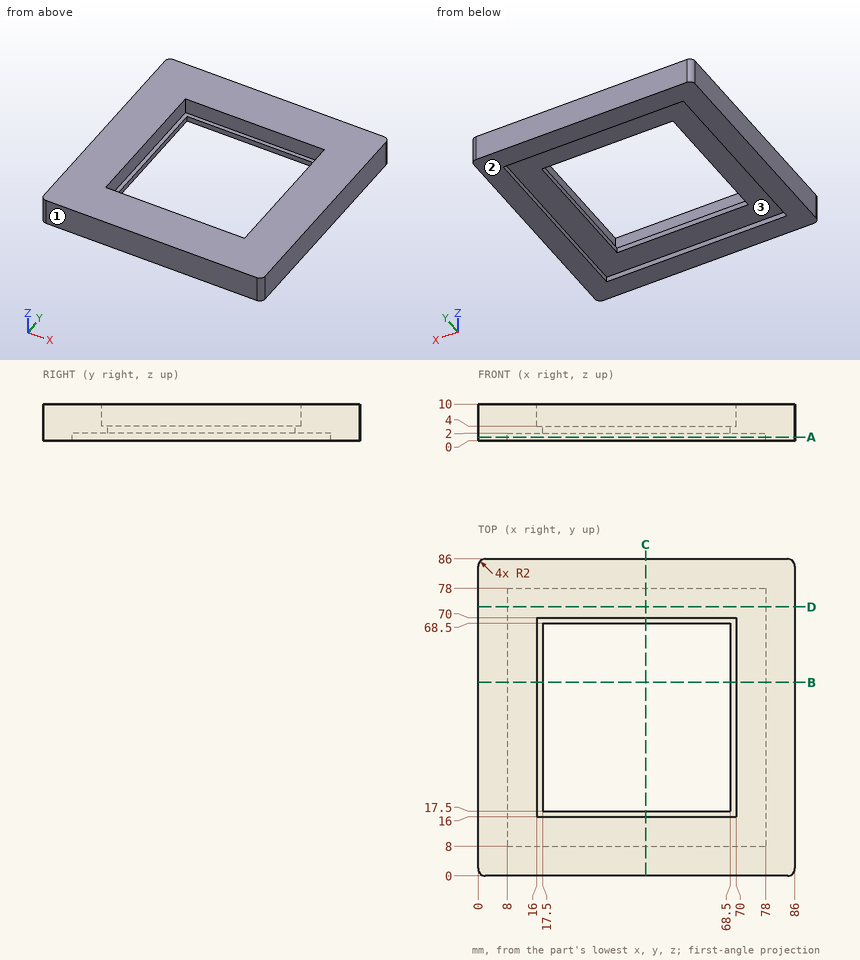
Geometry: see drawing. Coordinates: mm, zero at the bounding-box minimum. Coordinates: 2 decimals unless noted, no trailing zeros. Order: outer loops, then holes, each group sorted by start corner. A loop starts at its lowest first (then second) coordinate and runs counter-clockwise, first axis right, second up. Notation, with made-up numbers: M -10,-33 L 13,-33 A35 ccw 13,3 Z; hole C 38.5,46.25 d11. An arc over 180 degrees is marked long. Answer in a Markdown table with one row per item. Add a question column.
Q1. Line query: L1, parallel to Y at x = 50, z = 0.5; L2, parallel to Y at x = 51.5, z = 5.25. Output: solid intervals per line, ascending.
Q2. Section query D-D on y = 73. Return the cut outline in (x, z), and give its area (3 significant figures).
Q3. Section query B-B on y = 52.5. Return the cut outline in (x, z), and give its area (3 significant figures).
Q4. Contact query for a flat-ended pin moving along its axis: P1, Ø8, axis at x = 71.5, y = 57.5, coming from the -Z side. Output: stop coordinate, or through.
Q5. Mould query, pull axis Y, two halves, no side actions, for the marked faces 1, 2 and 3. Classes: released by +Y, released by -Y, zero draft, split by the parting line, or undercut.
Q6. Section query A-A on z = 1. Return the cut outline in (x, y), and give its area (3 significant figures).
Completed:
| question | item | result |
|---|---|---|
| 1 | L1 | y = 0 to 8, 78 to 86 |
| 1 | L2 | y = 0 to 16, 70 to 86 |
| 2 | outline | M 0,0 L 8,0 L 8,2 L 78,2 L 78,0 L 86,0 L 86,10 L 0,10 Z |
| 2 | area | 720 mm2 |
| 3 | outline | M 0,0 L 8,0 L 8,2 L 17.5,2 L 17.5,4 L 16,4 L 16,10 L 0,10 Z; M 68.5,2 L 78,2 L 78,0 L 86,0 L 86,10 L 70,10 L 70,4 L 68.5,4 Z |
| 3 | area | 294 mm2 |
| 4 | P1 | stops at z = 2 |
| 5 | face 1 | released by -Y |
| 5 | face 2 | zero draft |
| 5 | face 3 | undercut |
| 6 | outline | M 0,2 A2 ccw 2,0 L 84,0 A2 ccw 86,2 L 86,84 A2 ccw 84,86 L 2,86 A2 ccw 0,84 Z; hole M 8,8 L 78,8 L 78,78 L 8,78 Z |
| 6 | area | 2,490 mm2 |
